Job drawing, mm, ordinate dimensions from the low corner. One solid piece. A direction names the side the tool comes from. Coordinates: 2 decimals unless noted, no trailing zeros. Loops run counter-clockwise (first coordinate to the right, second up) from the corner with the lowest first, then second, coordinate; pieces in that order, holes last. Notation, with made-up numbers: (60.5, 6.5) -> (78.5, 6.5) arc R18 cw to (78.5, 15.5) -> close; hole circle Ø1 at (3, -7.5). An arc over 180 degrees is marked (long way). Answer as CSV lines item,"result". Start each with the question number.
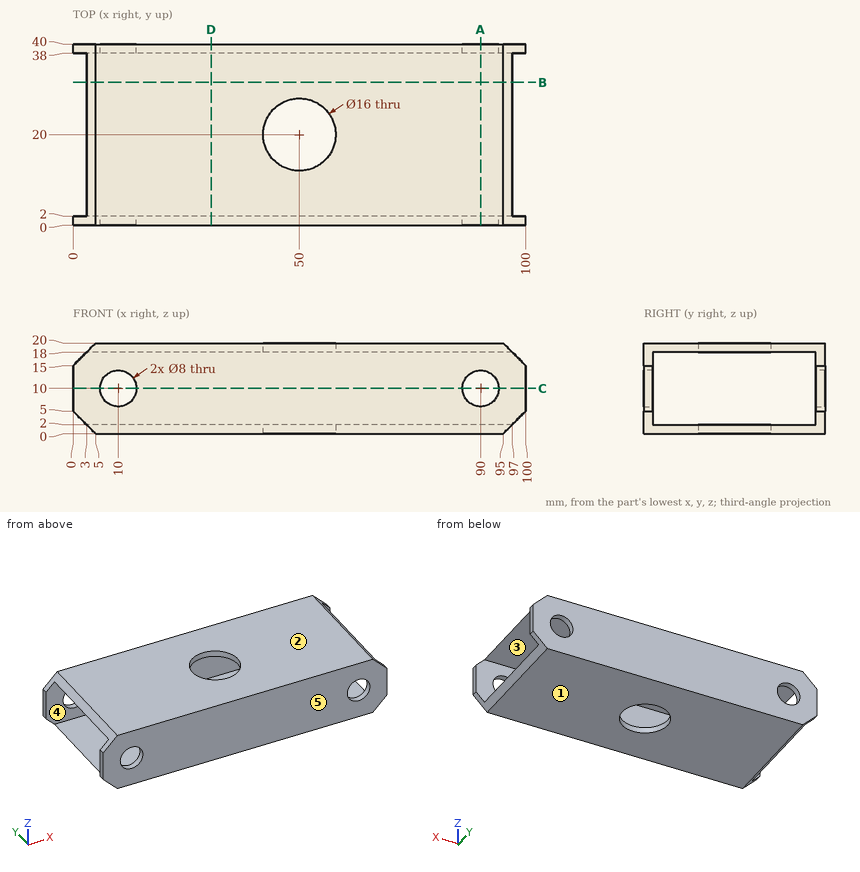
Q1. Saw through at A-A (x = 90). List the corners of the cut face in (y, z), and give its area (3 significant figures).
Q2. Saw through at C-C (z = 10). List the corners of the cut face in (x, y), and give its area (3 significant figures).
Q3. Probe probe 1 along X at (y, z) = (38.7, 10); probe 2 along Z at (x, y) = (29, 15); probe 3 along Y at (x, z) = (24, 2.5). List the from-to ranges inside material, lowest first. Write a range as from..to.
Q4. Saw through at D-D (x = 30.5). List the corners of the cut face in (y, z).
Q5. Which spindle directions (+Z, -Z, +X, -X, +Y, -Y) get a long thin tool onto all of the face, cutting with end or side? Do the marked faces 4 and 5. Say none if no direction does.
Q6. Two-plate mould, pull along Z, no slides. Class the marked faces 1, 2 and 3: pulls with the +Z half, pulls with the -Z half, needs draft (parallel to the pull), parting line crosses it, or undercut.
Q7. Saw through at B-B (y = 31.5). List the corners of the cut face in (x, z).
Q8. Pin check, flat tips, straight feed: pin 1 Ø5 at (x, z) = (10, 10) entering from +Y; pin 2 Ø6 at (x, z) = (30.5, 3) entering from -Y. Stop position of each tip, or through.
Ans:
1,outline,"(0, 0) -> (40, 0) -> (40, 6) -> (38, 6) -> (38, 2) -> (2, 2) -> (2, 6) -> (0, 6) -> close; (0, 14) -> (2, 14) -> (2, 18) -> (38, 18) -> (38, 14) -> (40, 14) -> (40, 20) -> (0, 20) -> close"
1,area,"192 mm²"
2,outline,"(0, 0) -> (6, 0) -> (6, 2) -> (0, 2) -> close; (0, 38) -> (6, 38) -> (6, 40) -> (0, 40) -> close; (14, 0) -> (86, 0) -> (86, 2) -> (14, 2) -> close; (14, 38) -> (86, 38) -> (86, 40) -> (14, 40) -> close; (94, 0) -> (100, 0) -> (100, 2) -> (94, 2) -> close; (94, 38) -> (100, 38) -> (100, 40) -> (94, 40) -> close"
2,area,"336 mm²"
3,probe 1,"x = 0..6, 14..86, 94..100"
3,probe 2,"z = 0..2, 18..20"
3,probe 3,"y = 0..2, 38..40"
4,outline,"(0, 0) -> (40, 0) -> (40, 20) -> (0, 20) -> close; hole (2, 2) -> (38, 2) -> (38, 18) -> (2, 18) -> close"
5,face 4,"+X, -X"
5,face 5,"+Z, -Z, +X, -X, -Y"
6,face 1,"pulls with the -Z half"
6,face 2,"pulls with the +Z half"
6,face 3,"undercut"
7,outline,"(3, 2) -> (5, 0) -> (95, 0) -> (97, 2) -> close; (3, 18) -> (97, 18) -> (95, 20) -> (5, 20) -> close"
8,pin 1,"passes through"
8,pin 2,"stops at y = 0"
